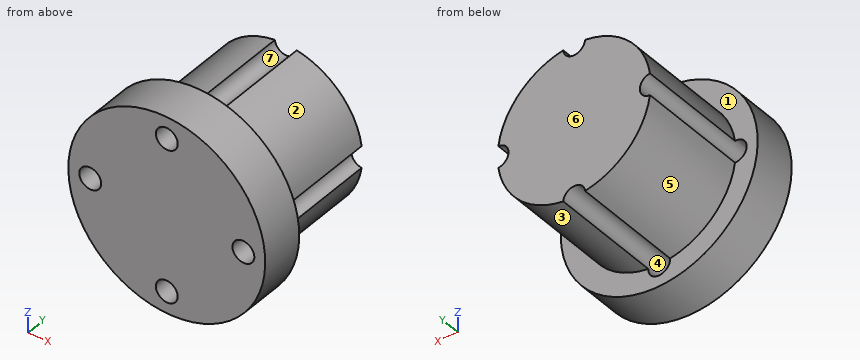
from build123d import *

# Parameters (mm, degrees)
SKETCH_1_R          = 9
EXTRUDE_1_DEPTH     = 14
SKETCH_2_R          = 1
CUT_EXTRUDE_1_DEPTH = 20
CUT_EXTRUDE_START   = -10
SKETCH_3_R          = 9
SKETCH_3_R_2        = 7
CUT_EXTRUDE_2_DEPTH = 10


with BuildPart() as part:
    # Эскиз1 → Бобышка-Вытянуть1 (new body)
    with BuildSketch(Plane(origin=(0, 0, 0), x_dir=(1, 0, 0), z_dir=(0, 1, 0))):
        with Locations(Location((0, 0, 0), (0, 0, 270))):
            Circle(SKETCH_1_R)
    extrude(amount=EXTRUDE_1_DEPTH)

    # Эскиз2 → Вырез-Вытянуть1 (cut)
    with BuildSketch(Plane(origin=(0, 14, 0), x_dir=(1, 0, 0), z_dir=(0, 1, 0))):
        with Locations(Location((0, 7, 0), (0, 0, 270))):
            Circle(SKETCH_2_R)
        with Locations(Location((7, 0, 0), (0, 0, 270))):
            Circle(SKETCH_2_R)
        with Locations(Location((-7, 0, 0), (0, 0, 270))):
            Circle(SKETCH_2_R)
        with Locations(Location((0, -7, 0), (0, 0, 270))):
            Circle(SKETCH_2_R)
    extrude(amount=-CUT_EXTRUDE_1_DEPTH, mode=Mode.SUBTRACT)

    # Эскиз3 → Вырез-Вытянуть2 (cut)
    with BuildSketch(Plane(origin=(0, 14, 0), x_dir=(1, 0, 0), z_dir=(0, 1, 0)).offset(CUT_EXTRUDE_START)):
        with Locations(Location((0, 0, 0), (0, 0, 270))):
            Circle(SKETCH_3_R)
        Circle(SKETCH_3_R_2, mode=Mode.SUBTRACT)
    extrude(amount=CUT_EXTRUDE_2_DEPTH, mode=Mode.SUBTRACT)


solid = part.part
Can you work these out from the model? Positions are in its coordinate system, mm. Face numbers are marked on the shaded views. A direction names the side the tool comes from. Round coordinates to 2 decimals unless told otherwise and drop trailing zeros. Write each loop counter-clockwise with the first axis right and the second up, starting at its lowest first coordinate (ties: lowest second). Pieces come first, ordered by that corner, then holes. Notation, with made-up numbers: (35, -16.75) -> (62, -16.75) arc R19 ccw to (62, 19.25) -> close; hole circle Ø3 at (-28.75, 79). An arc over 180 degrees is marked (long way). Use one line per item in the form item = value. Start each with the question number.
Q1. Imagine slicing it at C-C (y = 2). Please give me the cut outline in (x, z).
Q2. Imagine slicing it at A-A (z = 0). Please give me the cut outline in (x, y).
Q3. We'd pull the mould along Z, two halves only. Please class the marked faces 4, 5, 6 and 7: +Z half, -Z half, draft (parallel to the pull), parting line (faces both ways), or undercut.
Q4. I'm going to push flat-ended pins straight in: P1, Ø1, axis at y = 8, z = -4, coming from the -X side; P2, Ø6, axis at y = 6, z = -4, coming from the -X side; P3, Ø4, axis at x = 4.5, y = 10, coming from the -Z side. Where does each tip first touch, or does it pass through?
Q5. If I drill on probe 1 along Z at (x, y) = (-0.75, 1); probe 2 along Y at (x, z) = (7.75, -2.25); probe 3 along X at (y, z) = (8.75, 0), over which ranges is the centre line in solid material (lowest first)? Write a range as [from, to].
Q6. Imagine slicing it at B-B (x = 0). Please give me the cut outline in (y, z), then the cut area to 3 significant figures.
Q7. Imagine slicing it at D-D (z = 7.25). Please give me the cut outline in (x, y), then the cut area to 3 significant figures.
Q8. Which directions (+Z, -Z, +X, -X, +Y, -Y) give clear straight access to the entire face, cutting with the end or side of a thin tool? Please do the marked faces 1, 2 and 3.
Worked out:
q1.outline = circle Ø18 at (0, 0); hole circle Ø2 at (-7, 0); hole circle Ø2 at (0, -7); hole circle Ø2 at (0, 7); hole circle Ø2 at (7, 0)
q2.outline = (-9, 0) -> (-8, 0) -> (-8, 4) -> (-9, 4) -> close; (-6, 0) -> (6, 0) -> (6, 14) -> (-6, 14) -> close; (8, 0) -> (9, 0) -> (9, 4) -> (8, 4) -> close
q3.face_4 = undercut
q3.face_5 = -Z half
q3.face_6 = draft
q3.face_7 = undercut
q4.P1 = -6.06
q4.P2 = -8.83
q4.P3 = -6.54
q5.probe_1 = [-8.97, -7.66], [-6.34, 6.34], [7.66, 8.97]
q5.probe_2 = [0, 4]
q5.probe_3 = [-6, 6]
q6.outline = (0, -9) -> (4, -9) -> (4, -8) -> (0, -8) -> close; (0, -6) -> (14, -6) -> (14, 6) -> (0, 6) -> close; (0, 8) -> (4, 8) -> (4, 9) -> (0, 9) -> close
q6.area = 176 mm^2
q7.outline = (-5.33, 0) -> (-0.97, 0) -> (-0.97, 4) -> (-5.33, 4) -> close; (0.97, 0) -> (5.33, 0) -> (5.33, 4) -> (0.97, 4) -> close
q7.area = 34.9 mm^2
q8.face_1 = +Y
q8.face_2 = +Z, +X, +Y
q8.face_3 = -Z, +X, +Y
